The listing builds one solid part. Answer for the finished solid, in the listing's coordinates (mm). Face numbers are marked on the shaded views. A direction names the side the tool comes from. Round coordinates to 2 decimals unless told otherwise and drop trailing zeros. Loops run counter-clockwise (first coordinate to the right, second up) from the corner with the lowest first, then second, coordinate; pieces in that order, holes last. Notation, with made-up numbers: (-12.5, 45) -> (16.5, 45) arc R18 cw to (16.5, 80) -> close; hole circle Ø11 at (0, 54.5). An arc over 180 degrees is marked (long way). Use a Markdown table: item, result. Add a question column.
Q1. Consider line 1 (Z direction, x = -67, y = 57) (3 decimals); line 2 (X direction, y = 67, z = -28) (3 decimals); line 3 (X direction, y = 25, z = -105). Determine where each line is inside the solid, lowest interval first.
Q2. Given pin 1 Ø3 at (x, y) = (-107.5, 97.5) entering from +Z; pin 2 Ø12 at (x, z) = (-82, -34) entering from +Y (3 decimals); pin 3 Ø6 at (x, y) = (-25, 127) entering from -Z; pin 4 Ø6.5 at (x, y) = (47.6, 25.4) entering from +Z, each flat-ended and moving along its own axis, determine where each tip first touches the part or whether it passes through.
Q3. Section C-C on z = -56 is taken. Give the vertices of the cut face in (x, y) (3 decimals), then the cut area to 3 significant figures.
Q4. For a pull along X with two mould halves and no side action, classify the marked faces 1, 2 and 3 as released by +X, released by -X, zero draft, split by the parting line, or undercut.
Q5. Which of the six approach directions +Z, -Z, +X, -X, +Y, -Y give full straight-line access (tool end or side, diameter ignored) to the marked faces 4 and 5?
Q6. Section B-B on y = 25.4 is taken. Give the vertices of the cut face in (x, z) (3 decimals), then the cut area to 3 significant figures.
Q7. Section D-D on x = 119 is taken. Give the vertices of the cut face in (y, z) (3 decimals), then the cut area to 3 significant figures.
Q8. Section A-A on x = 47.6 is taken. Give the vertices of the cut face in (y, z) (3 decimals), then the cut area to 3 significant figures.
from build123d import *

# Parameters (mm, degrees)
SKETCH1_W               = 298.45
SKETCH1_H               = 209.55
BOSS_EXTRUDE1_DEPTH     = 3.175
SKETCH1_3_W             = 304.8
SKETCH1_3_H             = 215.9
SKETCH1_3_W_2           = 298.45
SKETCH1_3_H_2           = 209.55
BOSS_EXTRUDE2_DEPTH     = 177.8
SKETCH2_R               = 3.175
BOSS_EXTRUDE3_DEPTH     = 12.7
SKETCH2_3_R             = 4
CUT_EXTRUDE1_DEPTH      = 13.7
CUT_EXTRUDE1_DEPTH_BACK = 216.9


with BuildPart() as part:
    # Sketch1 → Boss-Extrude1 (new body)
    with BuildSketch(Plane(origin=(0, 0, 0), x_dir=(1, 0, 0), z_dir=(0, 1, 0))):
        Rectangle(SKETCH1_W, SKETCH1_H)
    extrude(amount=BOSS_EXTRUDE1_DEPTH)

    # Sketch1<3> → Boss-Extrude2 (add)
    with BuildSketch(Plane(origin=(0, 0, 0), x_dir=(1, 0, 0), z_dir=(0, 1, 0))):
        Rectangle(SKETCH1_3_W, SKETCH1_3_H)
        Rectangle(SKETCH1_3_W_2, SKETCH1_3_H_2, mode=Mode.SUBTRACT)
    extrude(amount=BOSS_EXTRUDE2_DEPTH)

    # Sketch2 → Boss-Extrude3 (add)
    with BuildSketch(Plane.XY.offset(107.95)):
        with Locations((25.4, 152.4)):
            Circle(SKETCH2_R)
    boss_extrude3 = extrude(amount=BOSS_EXTRUDE3_DEPTH)

    # Sketch2<3> → Cut-Extrude1 (cut, two sides)
    with BuildSketch(Plane.XY.offset(107.95)) as cut_extrude1_sk:
        with Locations((47.6, 25.4)):
            Circle(SKETCH2_3_R)
    extrude(amount=CUT_EXTRUDE1_DEPTH, mode=Mode.SUBTRACT)
    extrude(cut_extrude1_sk.sketch, amount=-CUT_EXTRUDE1_DEPTH_BACK, mode=Mode.SUBTRACT)

    # Mirror1: Boss-Extrude3 across plane
    add(boss_extrude3.mirror(Plane.XY))


solid = part.part
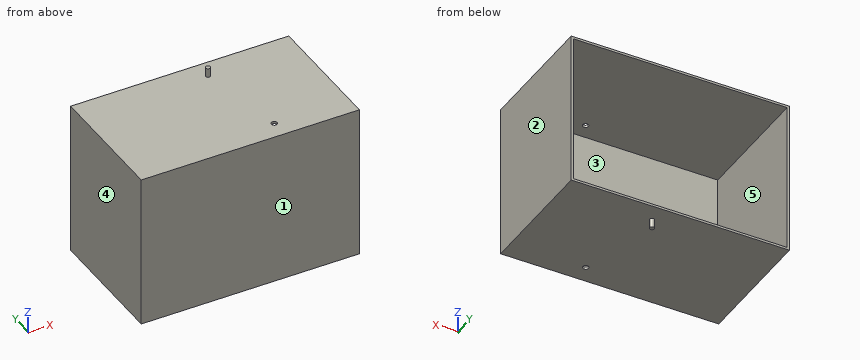
Checked values:
| question | item | result |
|---|---|---|
| 1 | line 1 | z = -107.95 to -104.775, 104.775 to 107.95 |
| 1 | line 2 | x = -152.4 to -149.225, 149.225 to 152.4 |
| 1 | line 3 | x = -152.4 to 43.62, 51.58 to 152.4 |
| 2 | pin 1 | stops at z = 107.95 |
| 2 | pin 2 | stops at y = 3.175 |
| 2 | pin 3 | stops at z = -107.95 |
| 2 | pin 4 | passes through |
| 3 | outline | (-152.4, 0) -> (152.4, 0) -> (152.4, 177.8) -> (149.225, 177.8) -> (149.225, 3.175) -> (-149.225, 3.175) -> (-149.225, 177.8) -> (-152.4, 177.8) -> close |
| 3 | area | 2,080 mm2 |
| 4 | face 1 | zero draft |
| 4 | face 2 | released by +X |
| 4 | face 3 | undercut |
| 5 | face 4 | +Z, -Z, -X, +Y, -Y |
| 5 | face 5 | +Y |
| 6 | outline | (-152.4, -107.95) -> (43.6, -107.95) -> (43.6, -104.775) -> (-149.225, -104.775) -> (-149.225, 104.775) -> (43.6, 104.775) -> (43.6, 107.95) -> (-152.4, 107.95) -> close; (51.6, -107.95) -> (152.4, -107.95) -> (152.4, 107.95) -> (51.6, 107.95) -> (51.6, 104.775) -> (149.225, 104.775) -> (149.225, -104.775) -> (51.6, -104.775) -> close |
| 6 | area | 3,220 mm2 |
| 7 | outline | (0, -107.95) -> (177.8, -107.95) -> (177.8, -104.775) -> (3.175, -104.775) -> (3.175, 104.775) -> (177.8, 104.775) -> (177.8, 107.95) -> (0, 107.95) -> close |
| 7 | area | 1,790 mm2 |
| 8 | outline | (0, -107.95) -> (21.4, -107.95) -> (21.4, -104.775) -> (3.175, -104.775) -> (3.175, 104.775) -> (21.4, 104.775) -> (21.4, 107.95) -> (0, 107.95) -> close; (29.4, -107.95) -> (177.8, -107.95) -> (177.8, -104.775) -> (29.4, -104.775) -> close; (29.4, 104.775) -> (177.8, 104.775) -> (177.8, 107.95) -> (29.4, 107.95) -> close |
| 8 | area | 1,740 mm2 |
